Input: part model. Units: mm. Frame: model coordinates. A direction names the side the tool comes from. Round coordinates to 2 decimals unless told otherwise and drop trailing zeros. Write each loop counter-clockwise with the first axis right and the second up, starting at its lowest first coordinate (ties: lowest second). Pieces come first, ordered by that corner, then holes. Notation, with made-up numbers: (0, 33.25) -> (30, 33.25) arc R24 ccw to (30, 65.25) -> close; hole circle Ø5 at (63, -11.5). An arc over 180 degrees is marked (long way). Write item = value, one per line. Start each with the question number.
```python
from build123d import *

# Parameters (mm, degrees)
SKETCH_2_R                 = 1.75
EXTRUDE_1_DEPTH            = 5
EXTRUDE_3_DEPTH            = 5
EXTRUDE_3_DEPTH_BACK       = 18
SKETCH_3_R                 = 6
SKETCH_3_R_2               = 4
CUT_EXTRUDE_2_DEPTH        = 25.166091947
CUT_EXTRUDE_2_DEPTH_BACK   = 25.166091947
SKETCH_7_R                 = 4
HOLE_START                 = -5.332682415
HOLE_WIZARD_M3_2_OUTLINE_R = 1.25
HOLE_WIZARD_M3_2_DEPTH     = 5.332682415
CHAMFER_2_SIZE             = 0.25
SKETCH_13_R                = 6
SKETCH_13_R_2              = 5.5
CUT_EXTRUDE_4_DEPTH        = 0.5


# Read off the part's stored shape, not the designer's step: M3 螺纹孔2
with BuildPart() as part:
    # 草图2 → 凸台-拉伸1 (new body)
    with BuildSketch(Plane(origin=(0, 0, 0), x_dir=(0, 0, -1), z_dir=(1, 0, 0))):
        with BuildLine():
            Line((-8, 11.489125293), (-8, -11.489125293))
            ThreePointArc((-8, -11.489125293), (0, -14), (8, -11.489125293))
            Line((8, -11.489125293), (8, 11.489125293))
            ThreePointArc((8, 11.489125293), (0, 14), (-8, 11.489125293))
        make_face()
        with Locations((0, 10)):
            Circle(SKETCH_2_R, mode=Mode.SUBTRACT)
        with Locations(Location((0, -10, 0), (0, 0, 180))):
            Circle(SKETCH_2_R, mode=Mode.SUBTRACT)
    extrude(amount=EXTRUDE_1_DEPTH)

    # 草图3 → 凸台-拉伸3 (add, two sides: drawn at the far end of the back side and taken through both)
    with BuildSketch(Plane.ZY.offset(-EXTRUDE_3_DEPTH_BACK)):
        Circle(SKETCH_3_R)
        Circle(SKETCH_3_R_2, mode=Mode.SUBTRACT)
    extrude(amount=EXTRUDE_3_DEPTH + EXTRUDE_3_DEPTH_BACK)

    # 草图7 → 切除-拉伸2 (cut, two sides: drawn at the far end of the back side and taken through both)
    with BuildSketch(Plane.ZY.offset(-CUT_EXTRUDE_2_DEPTH_BACK)):
        Circle(SKETCH_7_R)
    extrude(amount=CUT_EXTRUDE_2_DEPTH + CUT_EXTRUDE_2_DEPTH_BACK, mode=Mode.SUBTRACT)

    # M3 螺纹孔2 outline → M3 螺纹孔2 (cut)
    with BuildSketch(Plane.XY.offset(HOLE_START)):
        with Locations((14, -4)):
            Circle(HOLE_WIZARD_M3_2_OUTLINE_R)
        with Locations((14, 4)):
            Circle(HOLE_WIZARD_M3_2_OUTLINE_R)
    extrude(amount=HOLE_WIZARD_M3_2_DEPTH, mode=Mode.SUBTRACT)

    # 倒角2
    chamfer_2_edges = [part.edges().sort_by_distance(p)[0] for p in [
        (18, 0, -6),
    ]]
    chamfer(chamfer_2_edges, length=CHAMFER_2_SIZE)

    # 草图13 → 切除-拉伸4 (cut)
    with BuildSketch(Plane(origin=(5.5, 0, 0), x_dir=(0, 0, -1), z_dir=(1, 0, 0))):
        with Locations(Location((0, 0, 0), (0, 0, 180))):
            Circle(SKETCH_13_R)
        Circle(SKETCH_13_R_2, mode=Mode.SUBTRACT)
    extrude(amount=-CUT_EXTRUDE_4_DEPTH, mode=Mode.SUBTRACT)


solid = part.part
```
1. Section B-B (x = 1.5). Output: boundary loops of the cut face in (y, z).
2. Section A-A (y = -10). Output: boundary loops of the cut face in (x, z).
3. Section C-C (y = 0). Output: boundary loops of the cut face in (x, z).
4. Reachability of faces 4 (the cylindrical face through (-2, 0, -6)), 5 (the flat face through (14, -4.5, 0)), 6 (the cylindrical face through (11.71, -2.3, 5.54)), 7 (the cylindrical face through (5.25, -5.37, 1.19)) from +Z, -Z, +X, -X, +Y, -Y: full face, straight path, thin tool, end or side. Return the list, or none.
5. Line query: line 1 along Y through (x, z) = (4.25, 0); line 2 along X through (y, z) = (4, -1.55); line 3 along Y through (x, z) = (11.25, 0). Output: solid intervals per line, ascending.
6. Pin query (flat end, axial travel): P1, Ø5.5, axis at y = 10, z = 0, coming from the -X side; P2, Ø4, axis at x = 12.5, y = 3, coming from the +Z side; P3, Ø1, axis at x = 4.5, z = -4, coming from the -Y side. Return the tip coordinate at first contact, or that it passes through.
7. Section D-D (x = 16.25). Output: boundary loops of the cut face in (y, z).
8. Mould query, pull axis Z, two halves, no side actions, for faces 1 (the flat face through (2, 0, 8)), 2 (the cylindrical face through (13.01, -4.76, -2.7)), 3 (the cylindrical face through (2.465, -11.735, -0.228)). Classes: pulls with the +Z half, pulls with the -Z half, needs draft (parallel to the pull), parting line crosses it, or undercut.
Check sheet entries:
q1.outline = (-11.49, -8) -> (11.49, -8) arc R14 ccw to (11.49, 8) -> (-11.49, 8) arc R14 ccw to start; hole circle Ø3.5 at (-10, 0); hole circle Ø8 at (0, 0); hole circle Ø3.5 at (10, 0)
q2.outline = (0, -8) -> (5, -8) -> (5, -1.75) -> (0, -1.75) -> close; (0, 1.75) -> (5, 1.75) -> (5, 8) -> (0, 8) -> close
q3.outline = (-5, -6) -> (0, -6) -> (0, -8) -> (5, -8) -> (5, -5.5) -> (5.5, -5.5) -> (5.5, -6) -> (17.75, -6) -> (18, -5.75) -> (18, -4) -> (-5, -4) -> close; (-5, 4) -> (18, 4) -> (18, 5.75) -> (17.75, 6) -> (5.5, 6) -> (5.5, 5.5) -> (5, 5.5) -> (5, 8) -> (0, 8) -> (0, 6) -> (-5, 6) -> close
q4.face_4 = -X
q4.face_5 = -Z
q4.face_6 = +X
q4.face_7 = none
q5.line_1 = -14 to -11.75, -8.25 to -4, 4 to 8.25, 11.75 to 14
q5.line_2 = -5 to 12.75, 15.25 to 18
q5.line_3 = -6 to -4, 4 to 6
q6.P1 = 0
q6.P2 = 5.92
q6.P3 = -13.56
q7.outline = circle Ø12 at (0, 0); hole circle Ø8 at (0, 0)
q8.face_1 = pulls with the +Z half
q8.face_2 = needs draft
q8.face_3 = undercut
